```python
from build123d import *

# Parameters (mm, degrees)
F0_R     = 11.25
F1_DEPTH = 3
F2_DEPTH = 2
F3_DEPTH = 1.5
F4_R     = 11.25
F4_R_2   = 11
F5_DEPTH = 1


with BuildPart() as f1:
    # F0 (on Top) → F1 (new body)
    with BuildSketch(Plane.XY):
        Circle(F0_R)
        with BuildLine():
            ThreePointArc((7.7942286341, 4.5), (8.6933324366, 2.3293714059), (9, 0))
            ThreePointArc((9, 0), (8.6933324366, -2.3293714059), (7.7942286341, -4.5))
            ThreePointArc((7.7942286341, -4.5), (6.3639610307, -6.3639610307), (4.5, -7.7942286341))
            ThreePointArc((4.5, -7.7942286341), (2.3293714059, -8.6933324366), (0, -9))
            ThreePointArc((0, -9), (-2.3293714059, -8.6933324366), (-4.5, -7.7942286341))
            ThreePointArc((-4.5, -7.7942286341), (-6.3639610307, -6.3639610307), (-7.7942286341, -4.5))
            ThreePointArc((-7.7942286341, -4.5), (-8.6933324366, -2.3293714059), (-9, 0))
            ThreePointArc((-9, 0), (-8.6933324366, 2.3293714059), (-7.7942286341, 4.5))
            ThreePointArc((-7.7942286341, 4.5), (-6.3639610307, 6.3639610307), (-4.5, 7.7942286341))
            ThreePointArc((-4.5, 7.7942286341), (-2.3293714059, 8.6933324366), (0, 9))
            ThreePointArc((0, 9), (2.3293714059, 8.6933324366), (4.5, 7.7942286341))
            ThreePointArc((4.5, 7.7942286341), (6.3639610307, 6.3639610307), (7.7942286341, 4.5))
        make_face(mode=Mode.SUBTRACT)
    extrude(amount=F1_DEPTH)

    # F0 (on Top) → F2 (join)
    with BuildSketch(Plane.XY):
        with BuildLine():
            Line((-7.7942286341, 4.5), (-2.1650635095, 1.25))
            ThreePointArc((-2.1650635095, 1.25), (-1.767766953, 1.767766953), (-1.25, 2.1650635095))
            Line((-1.25, 2.1650635095), (-4.5, 7.7942286341))
            ThreePointArc((-4.5, 7.7942286341), (-6.3639610307, 6.3639610307), (-7.7942286341, 4.5))
        make_face()
        with BuildLine():
            Line((1.25, 2.1650635095), (4.5, 7.7942286341))
            ThreePointArc((4.5, 7.7942286341), (2.3293714059, 8.6933324366), (0, 9))
            Line((0, 9), (0, 2.5))
            ThreePointArc((0, 2.5), (0.6470476128, 2.4148145657), (1.25, 2.1650635095))
        make_face()
        with BuildLine():
            Line((2.5, 0), (9, 0))
            ThreePointArc((9, 0), (8.6933324366, 2.3293714059), (7.7942286341, 4.5))
            Line((7.7942286341, 4.5), (2.1650635095, 1.25))
            ThreePointArc((2.1650635095, 1.25), (2.4148145657, 0.6470476128), (2.5, 0))
        make_face()
        with BuildLine():
            ThreePointArc((4.5, -7.7942286341), (6.3639610307, -6.3639610307), (7.7942286341, -4.5))
            Line((7.7942286341, -4.5), (2.1650635095, -1.25))
            ThreePointArc((2.1650635095, -1.25), (1.767766953, -1.767766953), (1.25, -2.1650635095))
            Line((1.25, -2.1650635095), (4.5, -7.7942286341))
        make_face()
        with BuildLine():
            ThreePointArc((-4.5, -7.7942286341), (-2.3293714059, -8.6933324366), (0, -9))
            Line((0, -9), (0, -2.5))
            ThreePointArc((0, -2.5), (-0.6470476128, -2.4148145657), (-1.25, -2.1650635095))
            Line((-1.25, -2.1650635095), (-4.5, -7.7942286341))
        make_face()
        with BuildLine():
            ThreePointArc((-2.1650635095, -1.25), (-2.4148145657, -0.6470476128), (-2.5, 0))
            Line((-2.5, 0), (-9, 0))
            ThreePointArc((-9, 0), (-8.6933324366, -2.3293714059), (-7.7942286341, -4.5))
            Line((-7.7942286341, -4.5), (-2.1650635095, -1.25))
        make_face()
    extrude(amount=F2_DEPTH)

    # F0 (on Top) → F3 (join)
    with BuildSketch(Plane.XY):
        with BuildLine():
            Line((-9, 0), (-2.5, 0))
            ThreePointArc((-2.5, 0), (-2.4148145657, 0.6470476128), (-2.1650635095, 1.25))
            Line((-2.1650635095, 1.25), (-7.7942286341, 4.5))
            ThreePointArc((-7.7942286341, 4.5), (-8.6933324366, 2.3293714059), (-9, 0))
        make_face()
        with BuildLine():
            Line((0, 2.5), (0, 9))
            ThreePointArc((0, 9), (-2.3293714059, 8.6933324366), (-4.5, 7.7942286341))
            Line((-4.5, 7.7942286341), (-1.25, 2.1650635095))
            ThreePointArc((-1.25, 2.1650635095), (-0.6470476128, 2.4148145657), (0, 2.5))
        make_face()
        with BuildLine():
            Line((2.1650635095, 1.25), (7.7942286341, 4.5))
            ThreePointArc((7.7942286341, 4.5), (6.3639610307, 6.3639610307), (4.5, 7.7942286341))
            Line((4.5, 7.7942286341), (1.25, 2.1650635095))
            ThreePointArc((1.25, 2.1650635095), (1.767766953, 1.767766953), (2.1650635095, 1.25))
        make_face()
        with BuildLine():
            ThreePointArc((7.7942286341, -4.5), (8.6933324366, -2.3293714059), (9, 0))
            Line((9, 0), (2.5, 0))
            ThreePointArc((2.5, 0), (2.4148145657, -0.6470476128), (2.1650635095, -1.25))
            Line((2.1650635095, -1.25), (7.7942286341, -4.5))
        make_face()
        with BuildLine():
            ThreePointArc((0, -9), (2.3293714059, -8.6933324366), (4.5, -7.7942286341))
            Line((4.5, -7.7942286341), (1.25, -2.1650635095))
            ThreePointArc((1.25, -2.1650635095), (0.6470476128, -2.4148145657), (0, -2.5))
            Line((0, -2.5), (0, -9))
        make_face()
        with BuildLine():
            Line((-4.5, -7.7942286341), (-1.25, -2.1650635095))
            ThreePointArc((-1.25, -2.1650635095), (-1.767766953, -1.767766953), (-2.1650635095, -1.25))
            Line((-2.1650635095, -1.25), (-7.7942286341, -4.5))
            ThreePointArc((-7.7942286341, -4.5), (-6.3639610307, -6.3639610307), (-4.5, -7.7942286341))
        make_face()
    extrude(amount=F3_DEPTH)

    # F4 (on face) → F5 (cut)
    with BuildSketch(Plane(origin=(0, 0, 0), x_dir=(1, 0, 0), z_dir=(0, 0, -1))):
        Circle(F4_R)
        Circle(F4_R_2, mode=Mode.SUBTRACT)
    extrude(amount=-F5_DEPTH, mode=Mode.SUBTRACT)


solid = f1.part
```
Input: part model. Units: mm. Frame: model coordinates. A direction names the side the tool comes from. Give positions to 0.01 mm unless a question says otherwise; leave off trailing zeros. Write each loop counter-clockwise with the first axis right and the second up, starting at its lowest first coordinate (ties: lowest second). Pieces come first, ordered by that corner, then holes. Notation, with made-up numbers: (84, 62) - (114, 62) arc R26 cw to (114, 76) - close; hole circle Ø11 at (18, -13.75). An arc over 180 degrees is marked (long way). Write item = value, one per line. Start each with the question number.
1. Section query C-C, the plane y = 3. Output: boundary loops of the cut face in (x, z), then the cut area to 3 significant figures.
2. First-contact query: pin 1 Ø2 at (x, y) = (4.5, -3) entering from +Z; pin 2 Ø1.5 at (x, y) = (1, 1) entering from +Z; pin 3 Ø0.6 at (x, z) = (-6, 2) entering from +Y; pin 4 Ø1.3 at (x, y) = (2, -5) entering from +Z. Flat tips, straight axial feed; report the tip coordinate or a pass-through.
3. Mould query, pull axis Y, two halves, no side actions, for faces 1 (the flat face through (0, 3, 0)), 2 (the flat face through (-6, 2, 1.5)), 3 (the cylindrical face through (-2.38, 10.74, 0.49)). Classes: released by +Y, released by -Y, zero draft, split by the parting line, or undercut.
4. Ray query, L1, parallel to X at y = -4.75, z = 1.8; L2, parallel to X at y = 0, z = 0.5; L3, parallel to Y at x = 4.75, z = 1.55. Return the intervals inside material, ascending.
5. Section query B-B, the plane z = 2.5. Output: boundary loops of the cut face in (x, y), then the cut area to 3 significant figures.
6. Access query for faces 4 (the flat face through (6, 2, 2)), 5 (the flat face through (-5, 8, 3)). Directions: +Z, -Z, +X, -X, +Y, -Y. A direction counts if a zero-diameter tool reaches every point of the face in a straight line with its end or side. Return the directions, or none.
7. Section query A-A, the plane y = -0.5. Output: boundary loops of the cut face in (x, z).
Check sheet entries:
q1.outline = (-10.84, 1) - (-10.58, 1) - (-10.58, 0) - (10.58, 0) - (10.58, 1) - (10.84, 1) - (10.84, 3) - (8.49, 3) - (8.49, 2) - (5.2, 2) - (5.2, 1.5) - (1.73, 1.5) - (1.73, 2) - (0, 2) - (0, 1.5) - (-1.73, 1.5) - (-1.73, 2) - (-5.2, 2) - (-5.2, 1.5) - (-8.49, 1.5) - (-8.49, 3) - (-10.84, 3) - close
q1.area = 43.3 mm2
q2.pin_1 = 2
q2.pin_2 = through
q2.pin_3 = 9.7
q2.pin_4 = 1.5
q3.face_1 = zero draft
q3.face_2 = undercut
q3.face_3 = split by the parting line
q4.L1 = -10.2 to -7.64, -2.74 to 0, 2.74 to 10.2
q4.L2 = -11 to -2.5, 2.5 to 11
q4.L3 = -10.2 to -2.74, 0 to 2.74, 7.64 to 10.2
q5.outline = circle Ø22.5 at (0, 0); hole circle Ø18 at (0, 0)
q5.area = 143 mm2
q6.face_4 = +Z
q6.face_5 = +Z, +X, -X, +Y, -Y
q7.outline = (-11.24, 1) - (-10.99, 1) - (-10.99, 0) - (-2.45, 0) - (-2.45, 2) - (-8.99, 2) - (-8.99, 3) - (-11.24, 3) - close; (2.45, 0) - (10.99, 0) - (10.99, 1) - (11.24, 1) - (11.24, 3) - (8.99, 3) - (8.99, 1.5) - (2.45, 1.5) - close
